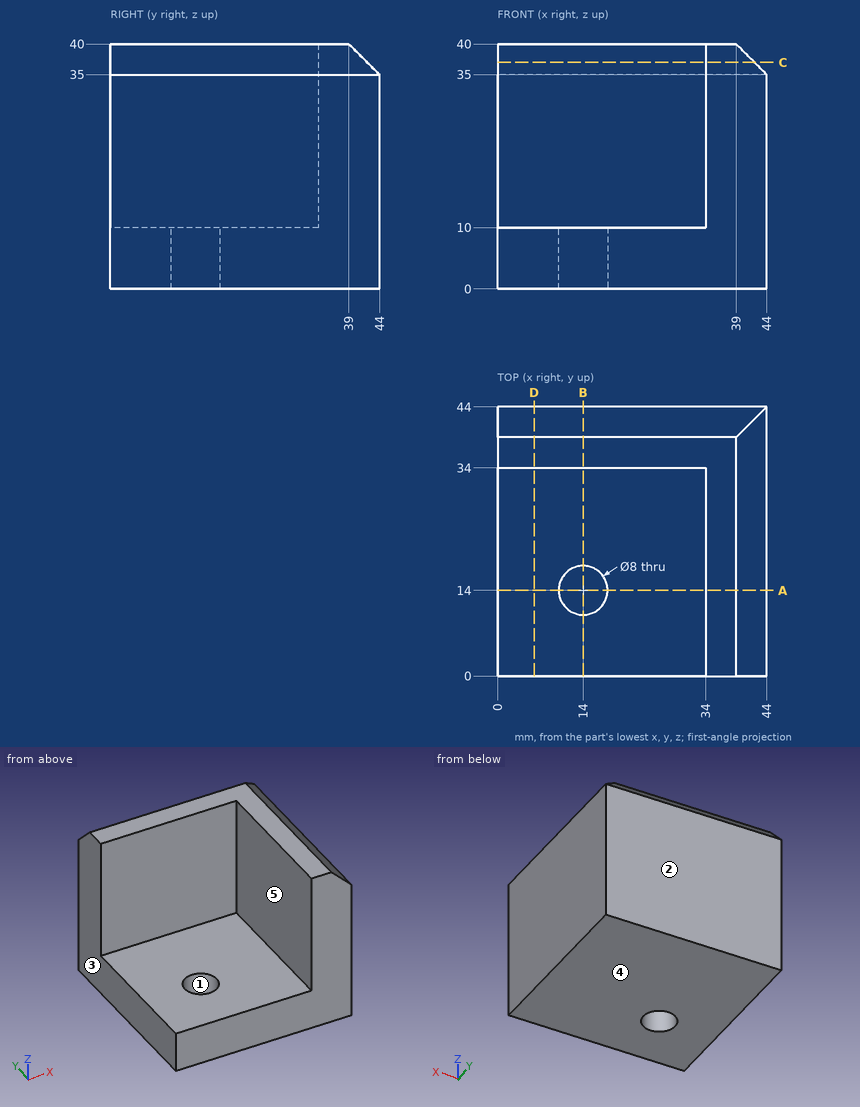
Design review of the part shown in the three views and the two pictorial views. Dimensions are in mm from the part's minimum x, y and z. A direction names the side the tool comes from. Coordinates: 2 decimals unless noted, no trailing zeros. Order: outer loops, then holes, each group sorted by start corner. A loop starts at its lowest first (then second) coordinate and runs counter-clockwise, first axis right, second up.
Item 1: Take a section at C-C, the plane z = 37. Write out the cut boundary in (x, y).
Item 2: Take a section at A-A, the plane y = 14. Write out the cut boundary in (x, z), then the cut area to 4 significant figures.
Item 3: For line 1 (Y direction, x = 14, z = 3.75); line 2 (Z direction, x = 20.5, y = 33); line 3 (Y direction, x = 31, z = 26.5), list the stretches that pass through material, from the lowest coordinate up.
Item 4: Take a section at D-D, the plane x = 6. Write out the cut boundary in (y, z), then the cut area to 4 significant figures.
Item 5: For pin 1 Ø4 at (y, z) = (7, 34.5) entering from -X; pin 2 Ø1.5 at (x, y) = (16.5, 29.5) entering from +Z; pin 3 Ø9 at (x, z) = (9, 30.5) entering from -Y; pin 4 Ø3 at (x, z) = (13, 5.5) entering from -Y, all flat-tipped, find the tip position at first contact; note any pin that passes through.
Item 6: For the marked faces 4 and 5, list the 3-axis set-ups (+Z, -Z, +X, -X, +Y, -Y) from which the entire face can be reached by the end or side of a thin tool; tool diameter is ignored.
Item 7: The part is to be moulded in two halves that separate along X. For the marked faces 1, 2 and 3, say which applies: pulls with the +X half, pulls with the -X half, needs draft (parallel to the pull), parting line crosses it, or undercut.
The answers:
1. outline: (0, 34) - (34, 34) - (34, 0) - (42, 0) - (42, 42) - (0, 42) - close
2. outline: (0, 0) - (10, 0) - (10, 10) - (0, 10) - close; (18, 0) - (44, 0) - (44, 35) - (39, 40) - (34, 40) - (34, 10) - (18, 10) - close
2. area: 647.5 mm2
3. line 1: y = 0 to 10, 18 to 44
3. line 2: z = 0 to 10
3. line 3: y = 34 to 44
4. outline: (0, 0) - (44, 0) - (44, 35) - (39, 40) - (34, 40) - (34, 10) - (0, 10) - close
4. area: 727.5 mm2
5. pin 1: stops at x = 34
5. pin 2: stops at z = 10
5. pin 3: stops at y = 34
5. pin 4: stops at y = 0
6. face 4: -Z, +X, -X, +Y, -Y
6. face 5: +Z, -X, -Y
7. face 1: undercut
7. face 2: needs draft
7. face 3: pulls with the -X half
